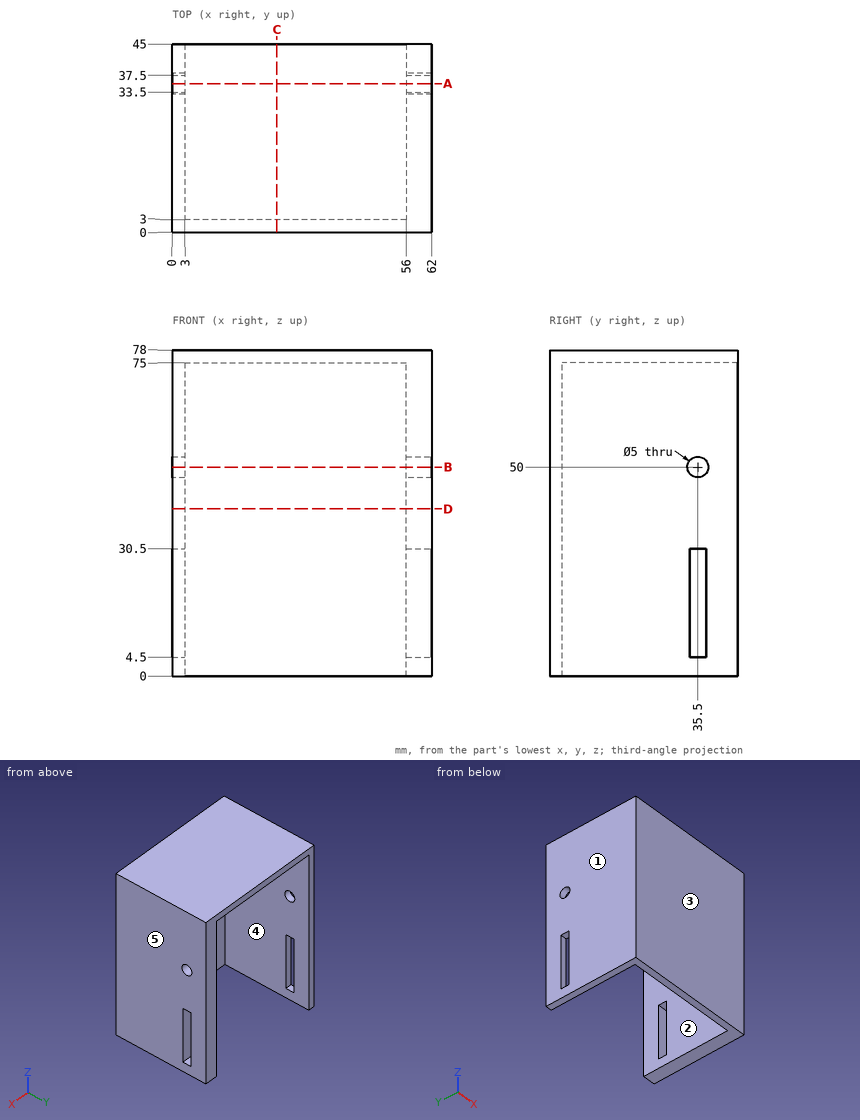
Geometry: see drawing. Coordinates: mm, zero at the bounding-box minimum. A direction names the side the tool comes from. Give positions to 0.01 mm unless a question says otherwise; leave off trailing zeros. Write each loop counter-clockwise with the first axis right and the second up, starting at its lowest first coordinate (ties: lowest second). Pieces come first, ordered by that corner, then holes. Notation, with made-up numbers: M 38.25,43.25 L 42.25,43.25 A24 cw 42.25,56.25 Z; hole C -28.75,49 d2. An arc over 180 degrees is marked long. Answer as a JSON object with one key per item and string values.
Q1. Contact query for flat-ended pins moving along their axis: P1, Ø4, axis at y = 35.5, z = 50, coming from the -X side; P2, Ø6, axis at x = 18, z = 30.5, coming from the +Y side; P3, Ø12.5, axis at x = 19.5, y = 20.5, coming from the -Z side. Output: stop coordinate, or through.
Geometry check:
{"P1": "passes through", "P2": "stops at y = 3", "P3": "stops at z = 75"}
Q2. Access query for the marked faces 1 and 2. Directions: +Z, -Z, +X, -X, +Y, -Y. A direction counts if a zero-diameter tool reaches every point of the face in a straight line with its end or side. Return the directions, or none.
Geometry check:
{"face 1": "+Z, -Z, -X, +Y, -Y", "face 2": "-Z, +Y"}
Q3. Cut plane D-D, the plane z = 40. Return the cut outline in (x, y), then the cut area to 3 significant figures.
Geometry check:
{"outline": "M 0,0 L 62,0 L 62,45 L 56,45 L 56,3 L 3,3 L 3,45 L 0,45 Z", "area": "564 mm^2"}
Q4. Cut plane C-C, the plane x = 25. Return the cut outline in (y, z), then the cut area to 3 significant figures.
Geometry check:
{"outline": "M 0,0 L 3,0 L 3,75 L 45,75 L 45,78 L 0,78 Z", "area": "360 mm^2"}
Q5. Cut plane A-A, the plane y = 35.5. Return the cut outline in (x, z), then the cut area to 3 significant figures.
Geometry check:
{"outline": "M 0,0 L 3,0 L 3,4.5 L 0,4.5 Z; M 0,30.5 L 3,30.5 L 3,47.5 L 0,47.5 Z; M 0,52.5 L 3,52.5 L 3,75 L 56,75 L 56,52.5 L 62,52.5 L 62,78 L 0,78 Z; M 56,0 L 62,0 L 62,4.5 L 56,4.5 Z; M 56,30.5 L 62,30.5 L 62,47.5 L 56,47.5 Z", "area": "582 mm^2"}
Q6. Mould query, pull axis X, two halves, no side actions, for the marked faces 3, 4 and 5. Classes: +X half, -X half, draft (parallel to the pull), parting line (faces both ways), or undercut.
Geometry check:
{"face 3": "draft", "face 4": "undercut", "face 5": "+X half"}
Q7. Ray query, line 1 along Z through (x, y) = (1, 35); line 2 along Y through (x, z) = (57.45, 50); line 3 along X through (y, z) = (15, 57.5). Return the intervals inside material, ascending.
Geometry check:
{"line 1": "z = 0 to 4.5, 30.5 to 47.55, 52.45 to 78", "line 2": "y = 0 to 33, 38 to 45", "line 3": "x = 0 to 3, 56 to 62"}
Q8. Cut plane B-B, the plane z = 50. Return the cut outline in (x, y), then the cut area to 3 significant figures.
Geometry check:
{"outline": "M 0,0 L 62,0 L 62,33 L 56,33 L 56,3 L 3,3 L 3,33 L 0,33 Z; M 0,38 L 3,38 L 3,45 L 0,45 Z; M 56,38 L 62,38 L 62,45 L 56,45 Z", "area": "519 mm^2"}
